The listing builds one solid part. Answer for the finished solid, in the listing's coordinates (mm). A direction names the side the tool comes from. Give positions to 0.01 mm unless a question says otherwise; leave off trailing zeros. Order: outer loops, then holes, each group sorted by start corner. A loop starts at its lowest first (then second) coordinate and runs counter-clockwise, first axis right, second up.
```python
from build123d import *

# Parameters (mm, degrees)
EXTRUDE_1_DEPTH          = 60
EXTRUDE_1_DEPTH_BACK     = 70
EXTRUDE_2_DEPTH          = 7.5
EXTRUDE_2_DEPTH_BACK     = 7.5
SKETCH_2_R               = 27
SKETCH_2_R_2             = 23.5
CUT_EXTRUDE_1_DEPTH      = 7.5
CUT_EXTRUDE_1_DEPTH_BACK = 7.5
SKETCH_3_R               = 24.5
SKETCH_4_R               = 24.5
EXTRUDE_3_DEPTH          = 3
EXTRUDE_4_DEPTH          = 2.58
SKETCH_6_R               = 1
CUT_EXTRUDE_2_DEPTH      = 3
SKETCH_7_R               = 1.5
CUT_EXTRUDE_3_DEPTH      = 5.58
CUT_EXTRUDE_4_DEPTH      = 97
CUT_EXTRUDE_5_DEPTH      = 1
CUT_EXTRUDE_5_DEPTH_BACK = 15
CUT_EXTRUDE_6_DEPTH      = 92.401586419
CUT_EXTRUDE_6_DEPTH_BACK = 7.5
SKETCH_10_R              = 2.5
EXTRUDE_5_DEPTH          = 4
EXTRUDE_5_DEPTH_BACK     = 4
EXTRUDE_6_DEPTH          = 4
EXTRUDE_6_DEPTH_BACK     = 4


with BuildPart() as part:
    # Sketch 1 → Extrude 1 (new, two sides: drawn at the far end of the back side and taken through both)
    with BuildSketch(Plane(origin=(0, 0, 0), x_dir=(0, 0, -1), z_dir=(1, 0, 0)).offset(-EXTRUDE_1_DEPTH_BACK)):
        Polygon((7.5, 0), (7.5, 15), (-7.5, 15), (-7.5, -15), (7.5, -15), align=None)
    extrude(amount=EXTRUDE_1_DEPTH + EXTRUDE_1_DEPTH_BACK)

    # Sketch 2 → Extrude 2 (add, two sides: drawn at the far end of the back side and taken through both)
    with BuildSketch(Plane.XY.offset(-EXTRUDE_2_DEPTH_BACK)):
        with Locations((60, 0)):
            Circle(SKETCH_2_R)
        with Locations((60, 0)):
            Circle(SKETCH_2_R_2, mode=Mode.SUBTRACT)
    extrude(amount=EXTRUDE_2_DEPTH + EXTRUDE_2_DEPTH_BACK)

    # Sketch 3 → Cut-Extrude 1 (cut, two sides: drawn at the far end of the back side and taken through both)
    with BuildSketch(Plane.XY.offset(-CUT_EXTRUDE_1_DEPTH_BACK)):
        with Locations((60, 0)):
            Circle(SKETCH_3_R)
    extrude(amount=CUT_EXTRUDE_1_DEPTH + CUT_EXTRUDE_1_DEPTH_BACK, mode=Mode.SUBTRACT)

    # Sketch 4 → Extrude 3 (add)
    with BuildSketch(Plane.XY.offset(7.5)):
        with Locations((60, 0)):
            Circle(SKETCH_4_R)
    extrude(amount=-EXTRUDE_3_DEPTH)

    # Sketch 5 → Extrude 4 (add)
    with BuildSketch(Plane(origin=(0, 0, 4.5), x_dir=(-1, 0, 0), z_dir=(0, 0, -1))):
        Polygon((-36.5, 0), (-36.5, 4), (-40.5, 4), (-45.5, 4), (-50.5, 4), (-50.5, 0), (-50.5, -4), (-36.5, -4), align=None)
    extrude(amount=EXTRUDE_4_DEPTH)

    # Sketch 6 → Cut-Extrude 2 (cut)
    with BuildSketch(Plane(origin=(0, 0, 4.5), x_dir=(-1, 0, 0), z_dir=(0, 0, -1))):
        with Locations((-60, 20.5)):
            Circle(SKETCH_6_R)
        with Locations((-60, -20.5)):
            Circle(SKETCH_6_R)
        with Locations((-45.894936823, 14.179111142)):
            Circle(SKETCH_6_R)
        with Locations(Location((-74.105063177, 14.179111142, 0), (0, 0, 180))):
            Circle(SKETCH_6_R)
        with Locations((-74.105063177, -14.179111142)):
            Circle(SKETCH_6_R)
        with Locations(Location((-45.894936823, -14.179111142, 0), (0, 0, 180))):
            Circle(SKETCH_6_R)
    extrude(amount=-CUT_EXTRUDE_2_DEPTH, mode=Mode.SUBTRACT)

    # Sketch 7 → Cut-Extrude 3 (cut)
    with BuildSketch(Plane(origin=(0, 0, 1.92), x_dir=(-1, 0, 0), z_dir=(0, 0, -1))):
        with Locations((-47.5, 0)):
            Circle(SKETCH_7_R)
        with Locations((-41, 0)):
            Circle(SKETCH_7_R)
    extrude(amount=-CUT_EXTRUDE_3_DEPTH, mode=Mode.SUBTRACT)

    # Sketch 8 → Cut-Extrude 4 (cut)
    with BuildSketch(Plane.ZY.offset(70)):
        Polygon((0, 15), (-3.75, 15), (-3.75, -15), (3.75, -15), (3.75, 15), align=None)
    extrude(amount=-CUT_EXTRUDE_4_DEPTH, mode=Mode.SUBTRACT)

    # Sketch 9 → Cut-Extrude 5 (cut, two sides: drawn at the far end of the back side and taken through both)
    with BuildSketch(Plane(origin=(36.5, 0, 0), x_dir=(0, 0, -1), z_dir=(1, 0, 0)).offset(-CUT_EXTRUDE_5_DEPTH_BACK)):
        Polygon((3.75, -9.1), (-4.5, -9.1), (-4.5, 9.1), (3.75, 9.1), (3.75, 0), align=None)
    extrude(amount=CUT_EXTRUDE_5_DEPTH + CUT_EXTRUDE_5_DEPTH_BACK, mode=Mode.SUBTRACT)

    # Sketch 10 → Cut-Extrude 6 (cut, two sides: drawn at the far end of the back side and taken through both)
    with BuildSketch(Plane.XY.offset(-CUT_EXTRUDE_6_DEPTH_BACK)):
        with BuildLine():
            Line((-60, 10), (-35, 15))
            Line((-35, 15), (-70, 15))
            Line((-70, 15), (-70, 8.3e-08))
            ThreePointArc((-70, 8.3e-08), (-67.071067782, 7.071067841), (-60, 10))
        make_face()
        with BuildLine():
            ThreePointArc((-60, -10), (-67.071067841, -7.071067782), (-70, 8.3e-08))
            Line((-70, 8.3e-08), (-70, -15))
            Line((-70, -15), (-35, -15))
            Line((-35, -15), (-60, -10))
        make_face()
        with Locations(Location((-60, 0, 0), (0, 0, 180))):
            Circle(SKETCH_10_R)
        with BuildLine():
            Line((-53.381882594, -6.370057829), (-47.910318504, -7.502760494))
            ThreePointArc((-47.910318504, -7.502760494), (-44.955257563, -6.500012961), (-44.393173811, -3.430493514))
            ThreePointArc((-44.393173811, -3.430493514), (-45, 0), (-44.393173811, 3.430493514))
            ThreePointArc((-44.393173811, 3.430493514), (-44.955257563, 6.500012961), (-47.910318504, 7.502760494))
            Line((-47.910318504, 7.502760494), (-53.381882594, 6.370057829))
            ThreePointArc((-53.381882594, 6.370057829), (-55.459731516, 4.768530579), (-55.483580368, 2.145216472))
            ThreePointArc((-55.483580368, 2.145216472), (-55, 0), (-55.483580368, -2.145216472))
            ThreePointArc((-55.483580368, -2.145216472), (-55.459731516, -4.768530579), (-53.381882594, -6.370057829))
        make_face()
        with Locations(Location((-35, 0, 0), (0, 0, 180))):
            Circle(SKETCH_10_R)
        with BuildLine():
            Line((-23.900962122, -10), (-21.539858023, -10))
            ThreePointArc((-21.539858023, -10), (-20.162567137, -9.674865726), (-19.076085186, -8.768113582))
            Line((-19.076085186, -8.768113582), (-8.695659254, 5.072454327))
            ThreePointArc((-8.695659254, 5.072454327), (-8.404850319, 8.29757484), (-11.159432091, 10))
            Line((-11.159432091, 10), (-23.900962122, 10))
            ThreePointArc((-23.900962122, 10), (-26.593808125, 8.414683944), (-26.514312819, 5.290851828))
            ThreePointArc((-26.514312819, 5.290851828), (-25, 0), (-26.514312819, -5.290851828))
            ThreePointArc((-26.514312819, -5.290851828), (-26.593808125, -8.414683944), (-23.900962122, -10))
        make_face()
        with BuildLine():
            Line((-0.923914814, 8.768113582), (-11.304340746, -5.072454327))
            ThreePointArc((-11.304340746, -5.072454327), (-11.595149681, -8.29757484), (-8.840567909, -10))
            Line((-8.840567909, -10), (5, -10))
            Line((5, -10), (5, 10))
            Line((5, 10), (1.539858023, 10))
            ThreePointArc((1.539858023, 10), (0.162567137, 9.674865726), (-0.923914814, 8.768113582))
        make_face()
        with BuildLine():
            Line((5, 10), (5, -10))
            Line((5, -10), (18.840567909, -10))
            ThreePointArc((18.840567909, -10), (21.595149681, -8.29757484), (21.304340746, -5.072454327))
            Line((21.304340746, -5.072454327), (10.923914814, 8.768113582))
            ThreePointArc((10.923914814, 8.768113582), (9.837432863, 9.674865726), (8.460141977, 10))
            Line((8.460141977, 10), (5, 10))
        make_face()
        with BuildLine():
            ThreePointArc((31.715728753, 10), (30, 0), (31.715728753, -10))
            Line((31.715728753, -10), (31.539858023, -10))
            ThreePointArc((31.539858023, -10), (30.162567137, -9.674865726), (29.076085186, -8.768113582))
            Line((29.076085186, -8.768113582), (18.695659254, 5.072454327))
            ThreePointArc((18.695659254, 5.072454327), (18.404850319, 8.29757484), (21.159432091, 10))
            Line((21.159432091, 10), (31.715728753, 10))
        make_face()
    extrude(amount=CUT_EXTRUDE_6_DEPTH + CUT_EXTRUDE_6_DEPTH_BACK, mode=Mode.SUBTRACT)

    # Sketch 11 → Extrude 5 (add, two sides: drawn at the far end of the back side and taken through both)
    with BuildSketch(Plane.XY.offset(-EXTRUDE_5_DEPTH_BACK)):
        with BuildLine():
            Line((-60, -7.5), (-34.519230769, -12.596153846))
            Line((-34.519230769, -12.596153846), (32.772497208, -12.596153846))
            ThreePointArc((32.772497208, -12.596153846), (33.368731111, -13.812151076), (34.019237886, -15))
            Line((34.019237886, -15), (-35, -15))
            Line((-35, -15), (-60, -10))
            ThreePointArc((-60, -10), (-62.588190451, -9.659258263), (-65, -8.660254038))
            Line((-65, -8.660254038), (-63.75, -6.495190528))
            ThreePointArc((-63.75, -6.495190528), (-61.941142838, -7.244443697), (-60, -7.5))
        make_face()
    extrude(amount=EXTRUDE_5_DEPTH + EXTRUDE_5_DEPTH_BACK)

    # Sketch 12 → Extrude 6 (add, two sides: drawn at the far end of the back side and taken through both)
    with BuildSketch(Plane.XY.offset(-EXTRUDE_6_DEPTH_BACK)):
        Polygon((13.695659254, 5.072454327), (21.304340746, -5.072454327), (26.304340746, -5.072454327), (18.695659254, 5.072454327), (15.018615082, 9.975179891), (10.018615082, 9.975179891), align=None)
        with BuildLine():
            Line((-19.076085186, -8.768113582), (-11.304340746, -8.768113582))
            ThreePointArc((-11.304340746, -8.768113582), (-11.920283955, -6.920283955), (-11.304340746, -5.072454327))
            Line((-11.304340746, -5.072454327), (-6.11412778, 1.847829627))
            Line((-6.11412778, 1.847829627), (-16.637943127, -5.517257503))
            Line((-16.637943127, -5.517257503), (-19.076085186, -8.768113582))
        make_face()
    extrude(amount=EXTRUDE_6_DEPTH + EXTRUDE_6_DEPTH_BACK)


solid = part.part
```
1) Given P1, Ø1.9, axis at x = 2, z = -6, coming from the +Y side; P2, Ø2.5, axis at x = 24, z = -0.5, coming from the -Y side; P3, Ø4, axis at x = -15, z = -1.5, coming from the +Y side, each flat-ended and moving along its own axis, determine where each tip first touches the part or whether it passes through.
Geometry says:
P1: stops at y = 15
P2: stops at y = -15
P3: stops at y = -2.97
2) For a pull along Y with two mould halves and no side action, classify faces 4 (the flat face through (-47.44, -10.01, -0.05)), 5 (the cylindrical face through (86.983, -0.965, -0.105)), 6 (the cylindrical face through (-11.858, -7.539, -0.105)), 7 (the flat face through (-17, 10, 6)) as +Y half, -Y half, draft (parallel to the pull), parting line (faces both ways), or undercut.
Geometry says:
face 4: +Y half
face 5: parting line
face 6: undercut
face 7: undercut
3) A tool of negligible diameter and unlimited length cuts with its end or side. For faces 1 (the flat face through (24, -6, 4.5)), 2 (the cylindrical face through (-61.968, -7.237, -0.053)), 3 (the flat face through (-50.608, 6.944, 5.599)), from which of +Z, -Z, +X, -X, +Y, -Y can it reach the whole face along a straight path? Write none if from no direction.
Geometry says:
face 1: none
face 2: +Y
face 3: +Z, -Z
4) Straight lines are drawn through the part: probe 1 along Y at (x, z) = (60, 6.9); probe 2 along Z at (x, y) = (20, -10); probe 3 along Y at (x, z) = (-35, 4.9). For each, find the intervals that lie inside material, in ascending order.
Geometry says:
probe 1: y = -27 to -21.5, -19.5 to 19.5, 21.5 to 27
probe 2: z = -7.5 to -3.75, 3.75 to 7.5
probe 3: y = -15 to -2.5, 2.5 to 15
5) Find section B-B (x = 41). Write down the section's boundary in (y, z).
Geometry says:
outline: (-19.18, -7.5) - (-15.47, -7.5) - (-15.47, 4.5) - (-4, 4.5) - (-4, 1.92) - (-1.5, 1.92) - (-1.5, 7.5) - (-19.18, 7.5) - close; (1.5, 1.92) - (4, 1.92) - (4, 4.5) - (15.47, 4.5) - (15.47, -7.5) - (19.18, -7.5) - (19.18, 7.5) - (1.5, 7.5) - close
6) Find section A-A (x = 6). Write down the section's boundary in (y, z), then the cut area to 3 significant figures.
Geometry says:
outline: (-15, -7.5) - (-10, -7.5) - (-10, -3.75) - (-12.6, -3.75) - (-12.6, 3.75) - (-10, 3.75) - (-10, 7.5) - (-15, 7.5) - close; (10, -7.5) - (15, -7.5) - (15, -3.75) - (10, -3.75) - close; (10, 3.75) - (15, 3.75) - (15, 7.5) - (10, 7.5) - close
area: 93.0 mm2
